Read the model definition and answer for the solid it produces. Units are mm, in the model's axes. A direction names the side the tool comes from. Coordinates: 2 decimals unless noted, no trailing zeros. Loops run counter-clockwise (first coordinate to the right, second up) from the corner with the lowest first, then second, coordinate; pieces in that order, holes last.
from build123d import *


with BuildPart() as part:
    # Esquisse1 → Révolution1 (revolve)
    with BuildSketch(Plane.XY):
        with BuildLine():
            Line((-2.5, 30.646225508), (-2.5, 27))
            Line((-2.5, 27), (-1.5, 26))
            Line((-1.5, 26), (-0.5, 26))
            Line((-0.5, 26), (-0.5, 23.6))
            Line((-0.5, 23.6), (2.5, 23.6))
            Line((2.5, 23.6), (2.5, 26.429629983))
            Line((2.5, 26.429629983), (0.646082423, 29.077298676))
            ThreePointArc((0.646082423, 29.077298676), (0.602504551, 29.575396025), (1.012080574, 29.862184243))
            Line((1.012080574, 29.862184243), (2.674311485, 30.007610604))
            Line((2.674311485, 30.007610604), (19.825688515, 30.007610604))
            Line((19.825688515, 30.007610604), (21.487919426, 29.862184243))
            ThreePointArc((21.487919426, 29.862184243), (21.897495449, 29.575396025), (21.853917577, 29.077298676))
            Line((21.853917577, 29.077298676), (20, 26.429629983))
            Line((20, 26.429629983), (20, 23.6))
            Line((20, 23.6), (23, 23.6))
            Line((23, 23.6), (23, 26))
            Line((23, 26), (24, 26))
            Line((24, 26), (25, 27))
            Line((25, 27), (25, 30.646225508))
            ThreePointArc((25, 30.646225508), (24.737277337, 31.321815716), (24.087155743, 31.642420206))
            Line((24.087155743, 31.642420206), (20, 32))
            Line((20, 32), (2.5, 32))
            Line((2.5, 32), (-1.587155743, 31.642420206))
            ThreePointArc((-1.587155743, 31.642420206), (-2.237277337, 31.321815716), (-2.5, 30.646225508))
        make_face()
    revolve(axis=Axis((10, 0, 0), (1, 0, 0)))


solid = part.part
Q1. Which of the six approach directions +Z, -Z, +X, -X, +Y, -Y give full straight-line access (tool end or side, diameter ignored) to faces 4 (the face through (2.5, 10, 22)), 5 (the face through (23, -6, -23)), 6 (the face through (-0.993, -20.633, -15.821))?
Findings below:
face 4: none
face 5: +X
face 6: -X
Q2. Determine the mould class of faces 1 (the face through (-0.5, 6, -23)), 2 (the face through (-2.5, 2.1, -27.1)), 3 (the face through (-1.389, -6.863, -30.907)) for opening direction Y: +Y half, -Y half, draft (parallel to the pull), parting line (faces both ways), or undercut.
Findings below:
face 1: undercut
face 2: draft
face 3: parting line
Q3. Straight lines are drawn through the part: probe 1 along Z at (x, y) = (15.75, 0); probe 2 along X at (y, z) = (-2.5, -24.5); probe 3 along Z at (x, y) = (1, -17). For each, find the intervals that lie inside material, in ascending order.
Findings below:
probe 1: z = -32 to -30.01, 30.01 to 32
probe 2: x = -0.5 to 2.5, 20 to 23
probe 3: z = -26.96 to -24.55, -22.96 to -16.37, 16.37 to 22.96, 24.55 to 26.96
Q4. A cutting plane is placed at A-A (x = 18.75). Give the vertices of the cut face in (y, z), then the cut area to 3 significant figures.
Findings below:
outline: circle Ø64 at (0, 0); hole circle Ø60.02 at (0, 0)
area: 388 mm2
Q5. Flat-ended cylindrical pins translate along their axes: pin 1 Ø2 at (x, z) = (21.5, 12) entering from +Y; pin 2 Ø12 at (x, z) = (9, 15) entering from -Y; pin 3 Ø10 at (x, z) = (1.5, 24.5) entering from -Y; pin 4 Ø16 at (y, z) = (-1.5, -8.5) entering from -X. Find the tip coordinate at first contact, or state that the pin passes through.
Findings below:
pin 1: stops at y = 29.92
pin 2: stops at y = -30.71
pin 3: stops at y = -25.3
pin 4: passes through
